Source: CAD feature listing. Evaluate the final solid. Frame: model axes, mm. Round coordinates to 2 decimals unless told otherwise and drop trailing zeros. Order: outer loops, then holes, each group sorted by start corner. A loop starts at its lowest first (then second) coordinate and runs counter-clockwise, first axis right, second up.
```python
from build123d import *

# Parameters (mm, degrees)
F1_DEPTH = 12.7
F2_R     = 12.7
F3_DEPTH = 25.4
F4_R     = 6.35
F5_DEPTH = 38.1
F7_DEPTH = 12.7


with BuildPart() as f1:
    # F0 (on Top) → F1 (new body)
    with BuildSketch(Plane.XY):
        with BuildLine():
            ThreePointArc((0, 25.4), (-12.7, 12.7), (0, 0))
            Line((0, 0), (0, 25.4))
        make_face()
        with BuildLine():
            ThreePointArc((12.7, 12.7), (8.9802561211, 3.7197438789), (0, 0))
            Line((0, 0), (63.5, 0))
            ThreePointArc((63.5, 0), (50.8, 12.7), (63.5, 25.4))
            Line((63.5, 25.4), (0, 25.4))
            ThreePointArc((0, 25.4), (8.9802561211, 21.6802561211), (12.7, 12.7))
        make_face()
        with BuildLine():
            Line((0, 25.4), (0, 0))
            ThreePointArc((0, 0), (8.9802561211, 3.7197438789), (12.7, 12.7))
            ThreePointArc((12.7, 12.7), (8.9802561211, 21.6802561211), (0, 25.4))
        make_face()
        with BuildLine():
            ThreePointArc((63.5, 25.4), (50.8, 12.7), (63.5, 0))
            Line((63.5, 0), (63.5, 25.4))
        make_face()
        with BuildLine():
            Line((63.5, 25.4), (63.5, 0))
            ThreePointArc((63.5, 0), (72.4802561211, 3.7197438789), (76.2, 12.7))
            ThreePointArc((76.2, 12.7), (72.4802561211, 21.6802561211), (63.5, 25.4))
        make_face()
    extrude(amount=F1_DEPTH)

    # F2 (on face) → F3 (join)
    with BuildSketch(Plane.XY.offset(12.7)):
        with Locations((0, 12.7)):
            Circle(F2_R)
    extrude(amount=F3_DEPTH)

    # F4 (on face) → F5 (cut)
    with BuildSketch(Plane.XY.offset(38.1)):
        with Locations((0, 12.7)):
            Circle(F4_R)
    extrude(amount=-F5_DEPTH, mode=Mode.SUBTRACT)

    # F6 (on face) → F7 (cut)
    with BuildSketch(Plane.XY.offset(12.7)):
        with BuildLine():
            ThreePointArc((38.257622641, 6.0399938281), (42.6467607914, 7.9533489918), (44.4519152548, 12.3880845024))
            ThreePointArc((44.4519152548, 12.3880845024), (42.5920433154, 16.878212563), (38.1019152548, 18.7380845024))
            Line((38.1019152548, 18.7380845024), (38.1019152548, 6.0380845024))
            Line((38.1019152548, 6.0380845024), (38.257622641, 6.0399938281))
        make_face()
        with BuildLine():
            ThreePointArc((38.1019152548, 18.7380845024), (42.5920433154, 16.878212563), (44.4519152548, 12.3880845024))
            ThreePointArc((44.4519152548, 12.3880845024), (42.6467607914, 7.9533489918), (38.257622641, 6.0399938281))
            Line((38.257622641, 6.0399938281), (63.5, 6.3495226148))
            Line((63.5, 6.3495226148), (63.4999941462, 6.35))
            ThreePointArc((63.4999941462, 6.35), (57.1504773494, 12.622140454), (63.3442867618, 19.0480905308))
            Line((63.3442867618, 19.0480905308), (38.1019152548, 18.7380845024))
        make_face()
        with BuildLine():
            Line((38.1019152548, 6.0380845024), (38.1019152548, 18.7380845024))
            ThreePointArc((38.1019152548, 18.7380845024), (31.7519152548, 12.3880845024), (38.1019152548, 6.0380845024))
        make_face()
        with BuildLine():
            ThreePointArc((38.1019152548, 6.0380845024), (38.1797748009, 6.0385618518), (38.257622641, 6.0399938281))
            Line((38.257622641, 6.0399938281), (38.1019152548, 6.0380845024))
        make_face()
        with BuildLine():
            Line((63.4999941462, 6.35), (63.3442867618, 19.0480905308))
            ThreePointArc((63.3442867618, 19.0480905308), (57.1504773494, 12.622140454), (63.4999941462, 6.35))
        make_face()
        with BuildLine():
            ThreePointArc((69.85, 12.7), (67.9347334157, 17.2448475807), (63.3442867618, 19.0480905308))
            Line((63.3442867618, 19.0480905308), (63.4999941462, 6.35))
            ThreePointArc((63.4999941462, 6.35), (67.9901259909, 8.2098698698), (69.85, 12.7))
        make_face()
    extrude(amount=-F7_DEPTH, mode=Mode.SUBTRACT)


solid = f1.part
```
1. Line query: line 1 along Y through (x, z) = (0, 9); line 2 along Z through (x, y) = (59, 2); line 3 along Y through (x, z) = (33, 12.5). Output: solid intervals per line, ascending.
2. Section C-C on z = 18.5. Return loops of the section in (x, y), plus the area to 3 significant figures.
3. Section D-D on y = 3. Return loops of the section in (x, z).
4. Section B-B on x = 4.5. Return loops of the section in (y, z), plus the area to 3 significant figures.
5. Pull-direction query (X, two-part tool) for faces 1 (the face through (-12.688, 13.258, 23.017)), 2 (the face through (3.414, 18.054, 19.317)), 3 (the face through (31, 13, 0)); classes: released by +X, released by -X, zero draft, split by the parting line, or undercut.
6. Section A-A on z = 5. State how many separate pieces and enclosed holes the cut face has, plus the area to 3 significant figures.
7. First-contact query: pin 1 (6 mm diameter, centred on y = 15.5, z = 13, fed in from -X); pin 2 (1.5 mm diameter, centred on x = 6, z = 33.5, fed in from -Y); pin 3 (1.5 mm diameter, centred on y = 22, z = 14.5, fed in from -X); pin 4 (3 mm diameter, centred on x = 36, y = 19.5, fed in from +Z). Flat tips, straight axial feed; report the tip coordinate or a pass-through.
Result:
1. line 1: y = 0 to 6.35, 19.05 to 25.4
1. line 2: z = 0 to 12.7
1. line 3: y = 0 to 8.61, 16.17 to 25.4
2. outline: circle Ø25.4 at (0, 12.7); hole circle Ø12.7 at (0, 12.7)
2. area: 380 mm2
3. outline: (-8.2, 0) - (71.7, 0) - (71.7, 12.7) - (8.2, 12.7) - (8.2, 38.1) - (-8.2, 38.1) - close
4. outline: (0, 0) - (8.22, 0) - (8.22, 38.1) - (0.82, 38.1) - (0.82, 12.7) - (0, 12.7) - close; (17.18, 0) - (25.4, 0) - (25.4, 12.7) - (24.58, 12.7) - (24.58, 38.1) - (17.18, 38.1) - close
4. area: 584 mm2
5. face 1: split by the parting line
5. face 2: undercut
5. face 3: zero draft
6. separate pieces: 1
6. enclosed holes: 2
6. area: 1,540 mm2
7. pin 1: stops at x = -12.7
7. pin 2: stops at y = 1.14
7. pin 3: stops at x = -9.39
7. pin 4: stops at z = 12.7
